Verification items for the finished model (mm, model axes). Give positions to 0.01 mm unless a question says otherwise; leave off trailing zeros. Loops run counter-clockwise (first coordinate to the right, second up) from the corner with the lowest first, then second, coordinate; pieces in that order, holes last. Notation, with made-up numbers: M -36.5,-17.5 L 14.5,-17.5 A15 ccw 14.5,-7.5 Z; hole C 33,-28 d11. An arc over 180 degrees is marked long. Use a Markdown table: item, result.
from build123d import *

# Parameters (mm, degrees)
SKETCH1_W           = 63.5
SKETCH1_H           = 190.5
BOSS_EXTRUDE1_DEPTH = 3.175
SKETCH3_R           = 2.0828
CUT_EXTRUDE2_DEPTH  = 526.850378691
SKETCH4_R           = 2.0828
CUT_EXTRUDE4_DEPTH  = 526.850378691
FILLET2_R           = 3.175
CUT_EXTRUDE5_DEPTH  = 526.850378691


with BuildPart() as part:
    # Sketch1 → Boss-Extrude1 (new body)
    with BuildSketch(Plane(origin=(0, 0, 0), x_dir=(1, 0, 0), z_dir=(0, 1, 0))):
        Polygon((-242.686835374, -133.432512515), (-242.686835374, -385.491221995), (-242.686835374, -387.371651362), (-191.886835374, -438.171651362), (239.913164626, -438.171651362), (290.713164626, -387.371651362), (290.713164626, -133.371651362), (176.413164626, -82.571651362), (176.413164626, -133.371651362), (74.813164626, -196.871651362), (-26.786835374, -196.871651362), (-128.386835374, -133.371651362), (-128.386835374, -82.571651362), (-242.686835374, -133.371651362), align=None)
        with Locations((233.563164626, -243.80020948)):
            Rectangle(SKETCH1_W, SKETCH1_H, mode=Mode.SUBTRACT)
        with Locations((-185.536835374, -243.80020948)):
            Rectangle(SKETCH1_W, SKETCH1_H, mode=Mode.SUBTRACT)
    extrude(amount=BOSS_EXTRUDE1_DEPTH)

    # Sketch3 → Cut-Extrude2 (cut, through all)
    with BuildSketch(Plane(origin=(0, 0, 0), x_dir=(1, 0, 0), z_dir=(0, 1, 0))):
        with Locations(Location((-114.278235374, -270.125471314, 0), (0, 0, 270))):
            Circle(SKETCH3_R)
        with Locations(Location((-143.449035374, -284.13540948, 0), (0, 0, 270))):
            Circle(SKETCH3_R)
        with Locations(Location((-114.278235374, -217.474947647, 0), (0, 0, 270))):
            Circle(SKETCH3_R)
        with Locations(Location((-143.449035374, -203.46500948, 0), (0, 0, 270))):
            Circle(SKETCH3_R)
        with Locations(Location((191.475364626, -284.13540948, 0), (0, 0, 270))):
            Circle(SKETCH3_R)
        with Locations(Location((162.304564626, -270.125471314, 0), (0, 0, 270))):
            Circle(SKETCH3_R)
        with Locations(Location((162.304564626, -217.474947647, 0), (0, 0, 270))):
            Circle(SKETCH3_R)
        with Locations(Location((191.475364626, -203.46500948, 0), (0, 0, 270))):
            Circle(SKETCH3_R)
    extrude(amount=CUT_EXTRUDE2_DEPTH, mode=Mode.SUBTRACT)

    # Sketch4 → Cut-Extrude4 (cut, through all)
    with BuildSketch(Plane(origin=(0, 0, 0), x_dir=(1, 0, 0), z_dir=(0, 1, 0))):
        with Locations(Location((111.325664626, -210.298576853, 0), (0, 0, 270))):
            Circle(SKETCH4_R)
        with Locations(Location((111.325664626, -413.498576853, 0), (0, 0, 270))):
            Circle(SKETCH4_R)
        with Locations(Location((-63.299335374, -413.498576853, 0), (0, 0, 90))):
            Circle(SKETCH4_R)
        with Locations(Location((-63.299335374, -210.298576853, 0), (0, 0, 90))):
            Circle(SKETCH4_R)
        with BuildLine():
            Line((-50.599335374, -216.648576853), (98.625664626, -216.648576853))
            Line((98.625664626, -216.648576853), (98.625664626, -232.523576853))
            ThreePointArc((98.625664626, -232.523576853), (108.150664626, -242.048576853), (98.625664626, -251.573576853))
            Line((98.625664626, -251.573576853), (98.625664626, -384.923576853))
            ThreePointArc((98.625664626, -384.923576853), (108.150664626, -394.448576853), (98.625664626, -403.973576853))
            Line((98.625664626, -403.973576853), (98.625664626, -419.848576853))
            Line((98.625664626, -419.848576853), (-50.599335374, -419.848576853))
            Line((-50.599335374, -419.848576853), (-50.599335374, -403.973576853))
            ThreePointArc((-50.599335374, -403.973576853), (-60.124335374, -394.448576853), (-50.599335374, -384.923576853))
            Line((-50.599335374, -384.923576853), (-50.599335374, -251.573576853))
            ThreePointArc((-50.599335374, -251.573576853), (-60.124335374, -242.048576853), (-50.599335374, -232.523576853))
            Line((-50.599335374, -232.523576853), (-50.599335374, -216.648576853))
        make_face()
    extrude(amount=CUT_EXTRUDE4_DEPTH, mode=Mode.SUBTRACT)

    # Fillet2
    fillet2_edges = [part.edges().sort_by_distance(p)[0] for p in [
        (98.625664626, 1.5875, 419.848576853),
        (98.625664626, 1.5875, 216.648576853),
        (-50.599335374, 1.5875, 216.648576853),
        (-50.599335374, 1.5875, 419.848576853),
    ]]
    fillet(fillet2_edges, radius=FILLET2_R)

    # Sketch6 → Cut-Extrude5 (cut, through all)
    with BuildSketch(Plane(origin=(0, 3.175, 0), x_dir=(1, 0, 0), z_dir=(0, 1, 0))):
        Polygon((-96.636835374, -438.171651362), (-191.886835374, -438.171651362), (-242.686835374, -387.371651362), (-242.686835374, -133.371651362), (-128.386835374, -82.571651362), (-128.386835374, -133.371651362), (-96.636835374, -153.215401362), align=None)
        Polygon((176.413164626, -133.371651362), (144.663164626, -153.215401362), (144.663164626, -438.171651362), (239.913164626, -438.171651362), (290.713164626, -387.371651362), (290.713164626, -133.371651362), (176.413164626, -82.571651362), align=None)
    extrude(amount=-CUT_EXTRUDE5_DEPTH, mode=Mode.SUBTRACT)


solid = part.part
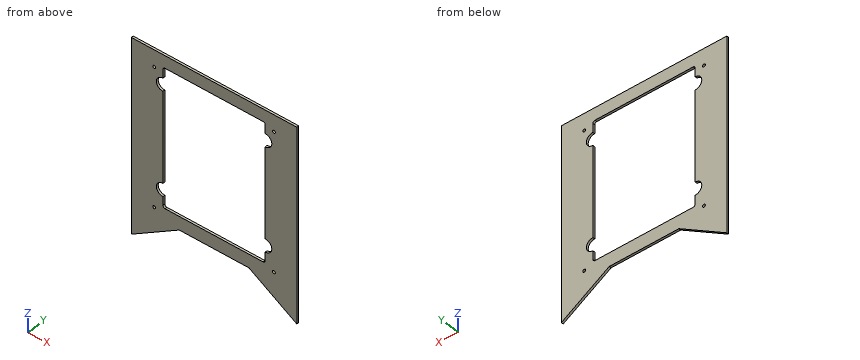
(1) Gauge pin test, flat ends, axial feed: P1, Ø1, axis at x = 6.5, y = 2, coming from the -Z side; P2, Ø1, axis at x = 109, y = 1.5, coming from the -Z side; P3, Ø5, axis at x = 111.33, z = 413.5, coming from the +Y side (3 decimals). Record the tip position at first contact, or that the pin passes through.
Results below:
| item | result |
|---|---|
| P1 | z = 196.87 |
| P2 | z = 175.19 |
| P3 | y = 3.175 |
(2) Cross-section at B-B on x = 36. Record the cut outline in (y, z) (3 decimals).
Results below:
| item | result |
|---|---|
| outline | M 0,196.872 L 3.175,196.872 L 3.175,216.649 L 0,216.649 Z; M 0,419.849 L 3.175,419.849 L 3.175,438.172 L 0,438.172 Z |
(3) Cross-section at A-A on z = 289. Record the cut outline in (x, y) (3 decimals).
Results below:
| item | result |
|---|---|
| outline | M -96.637,0 L -50.599,0 L -50.599,3.175 L -96.637,3.175 Z; M 98.626,0 L 144.663,0 L 144.663,3.175 L 98.626,3.175 Z |
(4) Material ranges on line 1 (Z direction, x = -62, y = 1.95); line 2 (X direction, y = 2.5, z = 302.5); line 3 (Z direction, x = 16, y = 2.9), recorded low to high.
Results below:
| item | result |
|---|---|
| line 1 | 174.86 to 208.67, 211.93 to 411.87, 415.13 to 438.17 |
| line 2 | -96.64 to -50.6, 98.63 to 144.66 |
| line 3 | 196.87 to 216.65, 419.85 to 438.17 |
(5) Cross-section at D-D on x = -77.5. Record the cut outline in (y, z) (3 decimals), then the cut area to 3 significant figures.
Results below:
| item | result |
|---|---|
| outline | M 0,165.176 L 3.175,165.176 L 3.175,438.172 L 0,438.172 Z |
| area | 867 mm^2 |
(6) Cross-section at C-C on y = 1.7. Record the cut outline in (x, z) (3 decimals).
Results below:
| item | result |
|---|---|
| outline | M -96.637,153.215 L -26.787,196.872 L 74.813,196.872 L 144.663,153.215 L 144.663,438.172 L -96.637,438.172 Z; hole C -63.299,210.299 d4.166; hole C -63.299,413.499 d4.166; hole M -50.599,219.824 A3.175 ccw -47.424,216.649 L 95.451,216.649 A3.175 ccw 98.626,219.824 L 98.626,232.524 A9.525 ccw 98.626,251.574 L 98.626,384.924 A9.525 ccw 98.626,403.974 L 98.626,416.674 A3.175 ccw 95.451,419.849 L -47.424,419.849 A3.175 ccw -50.599,416.674 L -50.599,403.974 A9.525 ccw -50.599,384.924 L -50.599,251.574 A9.525 ccw -50.599,232.524 Z; hole C 111.326,210.299 d4.166; hole C 111.326,413.499 d4.166 |
